from build123d import *

# Parameters (mm, degrees)
SKETCH1_W           = 71.12
SKETCH1_H           = 66.04
BOSS_EXTRUDE1_DEPTH = 20
FILLET1_R           = 4
SKETCH2_W           = 3.5
SKETCH2_H           = 7
BOSS_EXTRUDE2_DEPTH = 1.5


with BuildPart() as part:
    # Sketch1 → Boss-Extrude1 (new body)
    with BuildSketch(Plane(origin=(0, 0, 0), x_dir=(1, 0, 0), z_dir=(0, 1, 0))):
        Rectangle(SKETCH1_W, SKETCH1_H)
    extrude(amount=BOSS_EXTRUDE1_DEPTH)

    # Fillet1
    fillet1_edges = [part.edges().sort_by_distance(p)[0] for p in [
        (0, 20, 33.02),
        (0, 0, 33.02),
        (0, 0, -33.02),
        (0, 20, -33.02),
    ]]
    fillet(fillet1_edges, radius=FILLET1_R)

    # Sketch2 → Boss-Extrude2 (add)
    with BuildSketch(Plane(origin=(0, 20, 0), x_dir=(1, 0, 0), z_dir=(0, 1, 0))):
        with Locations((29.81, -19.82)):
            Rectangle(SKETCH2_W, SKETCH2_H)
    extrude(amount=BOSS_EXTRUDE2_DEPTH)


solid = part.part
Work out the finished part from the listing and answer in its coordinate system (mm). A direction names the side the tool comes from. Coordinates: 2 decimals unless noted, no trailing zeros. Loops run counter-clockwise (first coordinate to the right, second up) from the corner with the lowest first, then second, coordinate; pieces in that order, holes last. Notation, with made-up numbers: (36, 60) -> (77, 60) arc R15 cw to (77, 81) -> close; hole circle Ø3 at (5, 39.25). An arc over 180 degrees is marked (long way). Write each question's results on one line, items separated by ' | '. Start each with the question number.
1) Find section A-A on x = 5. Determine the outline of the cut face in (y, z).
2) For faces 1 (the flat face through (31.56, 21, 20)), 2 (the flat face through (28.06, 21, 20)), 3 (the flat face through (30, 21, 23.32)), determine the directions among +Z, -Z, +X, -X, +Y, -Y from which every point of the face is accessible in a straight line to the end or side of a thin tool.
3) Find section B-B on z = 2. Determine the outline of the cut face in (x, y).
4) Flat-ended cylindrical pins translate along their axes: P1, Ø1, axis at x = -27.5, y = 17.5, coming from the +Z side; P2, Ø6, axis at x = 22, z = 8, coming from the +Y side; P3, Ø0.8, axis at y = 21, z = 19, coming from the -X side. Find the tip coordinate at first contact, or state that the pin passes through.
5) Find section C-C on y = 1.75. Determine the outline of the cut face in (x, z).
6) Consider line 1 along Y through (x, z) = (-15, -2); line 2 along Z through (x, y) = (6, 3.5); line 3 along Z through (x, y) = (7, 2). Determine where each line is inside the solid, lowest interval first.
Response values:
1) outline: (0, -29.02) arc R4 ccw to (4, -33.02) -> (16, -33.02) arc R4 ccw to (20, -29.02) -> (20, 29.02) arc R4 ccw to (16, 33.02) -> (4, 33.02) arc R4 ccw to (0, 29.02) -> close
2) face 1: +Z, -Z, +X, +Y | face 2: +Z, -Z, -X, +Y | face 3: +Z, +X, -X, +Y
3) outline: (-35.56, 0) -> (35.56, 0) -> (35.56, 20) -> (-35.56, 20) -> close
4) P1: stops at z = 32.89 | P2: stops at y = 20 | P3: stops at x = 28.06
5) outline: (-35.56, -32.33) -> (35.56, -32.33) -> (35.56, 32.33) -> (-35.56, 32.33) -> close
6) line 1: y = 0 to 20 | line 2: z = -32.99 to 32.99 | line 3: z = -32.48 to 32.48
